```python
from build123d import *

# Parameters (mm, degrees)
SKETCH1_W           = 9.397838239
SKETCH1_H           = 22.517705726
SKETCH1_R           = 2.425
SKETCH1_W_2         = 4
SKETCH1_H_2         = 3
BOSS_EXTRUDE1_DEPTH = 3
FILLET1_R           = 1


with BuildPart() as part:
    # Sketch1 → Boss-Extrude1 (new body)
    with BuildSketch(Plane(origin=(0, 0, 0), x_dir=(0, 0, -1), z_dir=(1, 0, 0))):
        with Locations((-0.280633356, -0.315954963)):
            Rectangle(SKETCH1_W, SKETCH1_H)
        with Locations((-0.280633356, -0.315954963)):
            Circle(SKETCH1_R, mode=Mode.SUBTRACT)
        with Locations((-0.315702717, -6.918104791)):
            Rectangle(SKETCH1_W_2, SKETCH1_H_2, mode=Mode.SUBTRACT)
        with Locations((-0.315702717, 6.831895209)):
            Rectangle(SKETCH1_W_2, SKETCH1_H_2, mode=Mode.SUBTRACT)
    extrude(amount=BOSS_EXTRUDE1_DEPTH)

    # Fillet1
    fillet1_edges = [part.edges().sort_by_distance(p)[0] for p in [
        (1.5, 10.9428979, 4.979552475),
        (1.5, 10.9428979, -4.418285764),
        (1.5, -11.574807826, -4.418285764),
        (1.5, -11.574807826, 4.979552475),
    ]]
    fillet(fillet1_edges, radius=FILLET1_R)


solid = part.part
```
Source: CAD feature listing. Evaluate the final solid. Frame: model axes, mm. A direction names the side the tool comes from. Coordinates: 2 decimals unless noted, no trailing zeros. Write each loop counter-clockwise with the first axis right and the second up, starting at its lowest first coordinate (ties: lowest second). Pieces come first, ordered by that corner, then holes. Notation, with made-up numbers: M -31,65.25 L -11,65.25 A20 cw -11,101.25 Z; hole C -3.5,80 d4. An arc over 180 degrees is marked long. Answer as a JSON object with one key per item and string values.
1. Cut plane C-C on x = 1. Output: boundary loops of the cut face in (y, z) (3 decimals).
Evaluation:
{"outline": "M -11.575,-3.418 A1 ccw -10.575,-4.418 L 9.943,-4.418 A1 ccw 10.943,-3.418 L 10.943,3.98 A1 ccw 9.943,4.98 L -10.575,4.98 A1 ccw -11.575,3.98 Z; hole M -8.418,-1.684 L -5.418,-1.684 L -5.418,2.316 L -8.418,2.316 Z; hole C -0.316,0.281 d4.85; hole M 5.332,-1.684 L 8.332,-1.684 L 8.332,2.316 L 5.332,2.316 Z"}
2. Cut plane B-B on y = 0.25. Output: boundary loops of the cut face in (x, z), plus the area to 3 significant figures.
Evaluation:
{"outline": "M 0,-4.42 L 3,-4.42 L 3,-2.08 L 0,-2.08 Z; M 0,2.64 L 3,2.64 L 3,4.98 L 0,4.98 Z", "area": "14.0 mm^2"}
3. Cut plane A-A on z = -0.5. Output: boundary loops of the cut face in (x, y), plus the area to 3 significant figures.
Evaluation:
{"outline": "M 0,-11.57 L 3,-11.57 L 3,-8.42 L 0,-8.42 Z; M 0,-5.42 L 3,-5.42 L 3,-2.61 L 0,-2.61 Z; M 0,1.98 L 3,1.98 L 3,5.33 L 0,5.33 Z; M 0,8.33 L 3,8.33 L 3,10.94 L 0,10.94 Z", "area": "35.8 mm^2"}
4. Access query for faces 4 (the flat face through (1, 5.332, 0)), 5 (the cylindrical face through (1.521, 10.658, -4.118)). Directions: +Z, -Z, +X, -X, +Y, -Y. A direction counts if a zero-diameter tool reaches every point of the face in a straight line with its end or side. Return the directions, or none.
Evaluation:
{"face 4": "+X, -X", "face 5": "-Z, +X, -X, +Y"}
5. Draft query along Z for faces 1 (the flat face through (1, -7, 2.316)), 2 (the cylindrical face through (1.52, -11.29, -4.12)), 3 (the cylindrical face through (1.521, 10.642, 4.694)). Return one class per face: released by +Z, released by -Z, zero draft, split by the parting line, or undercut.
Evaluation:
{"face 1": "undercut", "face 2": "released by -Z", "face 3": "released by +Z"}
6. Ray query, L1, parallel to Y at x = 2.8, z = 0.25; L2, parallel to Z at x = 1.3, y = 7.75; L3, parallel to Y at x = 2.85, z = -1.25. Return the intervals inside material, ascending.
Evaluation:
{"L1": "-11.57 to -8.42, -5.42 to -2.74, 2.11 to 5.33, 8.33 to 10.94", "L2": "-4.42 to -1.68, 2.32 to 4.98", "L3": "-11.57 to -8.42, -5.42 to -2.2, 1.56 to 5.33, 8.33 to 10.94"}
7. Cut plane D-D on z = 2. Output: boundary loops of the cut face in (x, y).
Evaluation:
{"outline": "M 0,-11.57 L 3,-11.57 L 3,-8.42 L 0,-8.42 Z; M 0,-5.42 L 3,-5.42 L 3,-2.03 L 0,-2.03 Z; M 0,1.39 L 3,1.39 L 3,5.33 L 0,5.33 Z; M 0,8.33 L 3,8.33 L 3,10.94 L 0,10.94 Z"}
